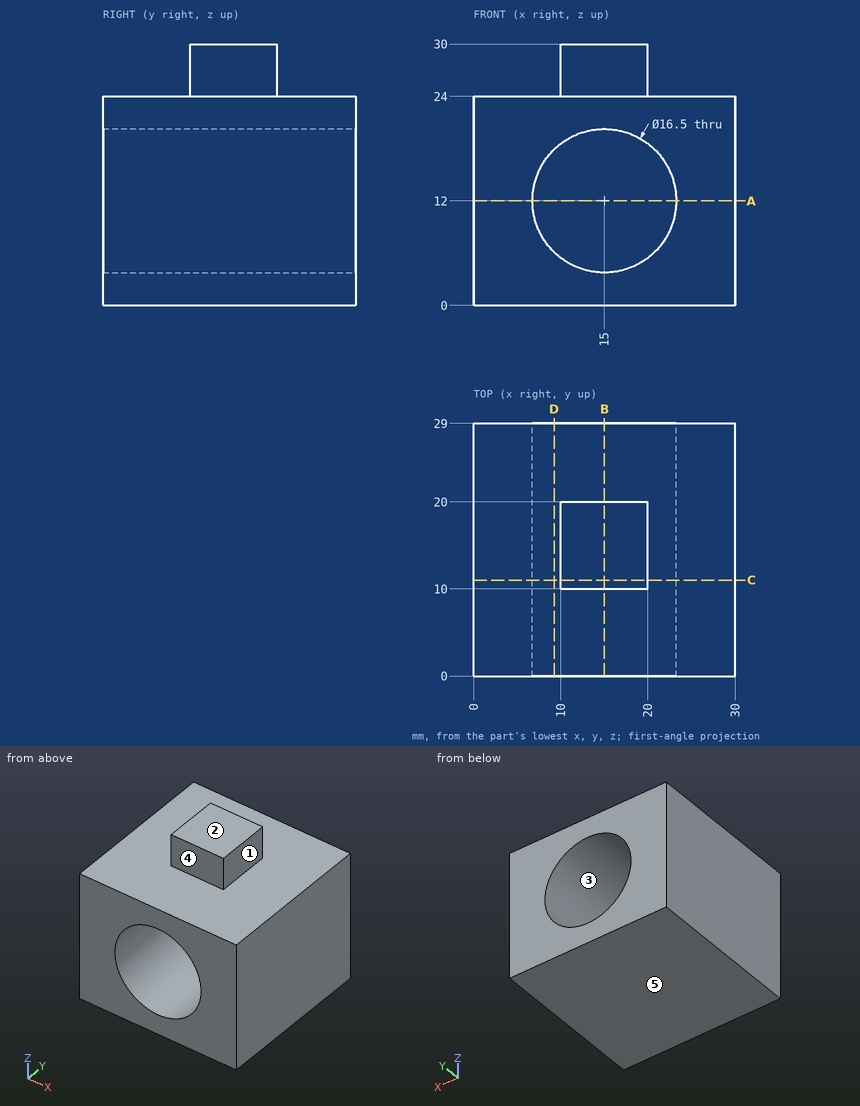
Geometry check sheet. Reference: drawing and pictorial views, mm from the part's lowest x, y, z. A direction names the side the tool comes from. Coordinates: 2 decimals unless noted, no trailing zeros. Loops run counter-clockwise (first coordinate to the right, second up) from the corner with the lowest first, then second, coordinate; pieces in that order, holes last. Notation, with made-up numbers: (0, 55.5) -> (53, 55.5) arc R30 cw to (53, 91.5) -> close; hole circle Ø1 at (12.5, 78). An arc over 180 degrees is marked (long way). Put each result on its own line as item: value.
1) Tool access check on the marked faces 1 and 2. Record the directions out of +Z, -Z, +X, -X, +Y, -Y that give a thin tool (end or side, any length) a straight path to the whole face; none if there is none.
Result set:
face 1: +Z, +X, +Y, -Y
face 2: +Z, +X, -X, +Y, -Y
2) Gauge pin test, flat ends, axial feed: pin 1 Ø1.8 at (y, z) = (17, 26) entering from -X; pin 2 Ø5 at (x, z) = (19.5, 14.5) entering from +Y; pin 3 Ø6.5 at (x, z) = (15.5, 27.5) entering from -Y; pin 4 Ø1.8 at (x, z) = (14, 27.5) entering from +Y. Record the tip position at first contact, or that the pin passes through.
Result set:
pin 1: stops at x = 10
pin 2: passes through
pin 3: stops at y = 10
pin 4: stops at y = 20
3) Thickness scan on line 1 (X direction, y = 23, z = 12); line 2 (X direction, y = 5.5, z = 18.75); line 3 (Z direction, x = 19.75, y = 27). Record the ranges inside material, lowest first.
Result set:
line 1: x = 0 to 6.75, 23.25 to 30
line 2: x = 0 to 10.26, 19.74 to 30
line 3: z = 0 to 5.25, 18.75 to 24
4) Cross-section at A-A on z = 12. Record the boundary of the cut face in (x, y), plus the area to 4 significant figures.
Result set:
outline: (0, 0) -> (6.75, 0) -> (6.75, 29) -> (0, 29) -> close; (23.25, 0) -> (30, 0) -> (30, 29) -> (23.25, 29) -> close
area: 391.5 mm^2
5) Cross-section at C-C on y = 11. Record the boundary of the cut face in (x, z).
Result set:
outline: (0, 0) -> (30, 0) -> (30, 24) -> (20, 24) -> (20, 30) -> (10, 30) -> (10, 24) -> (0, 24) -> close; hole circle Ø16.5 at (15, 12)
6) Release check for a two-part mould opening along Z. For the marked faces 3, 4 and 5 record: released by +Z, released by -Z, zero draft, split by the parting line, or undercut.
Result set:
face 3: undercut
face 4: zero draft
face 5: released by -Z
7) Cross-section at B-B on x = 15. Record the boundary of the cut face in (y, z), plus the area to 4 significant figures.
Result set:
outline: (0, 0) -> (29, 0) -> (29, 3.75) -> (0, 3.75) -> close; (0, 20.25) -> (29, 20.25) -> (29, 24) -> (20, 24) -> (20, 30) -> (10, 30) -> (10, 24) -> (0, 24) -> close
area: 277.5 mm^2
8) Cross-section at D-D on x = 9.25. Record the boundary of the cut face in (y, z), plus the area to 3 significant figures.
Result set:
outline: (0, 0) -> (29, 0) -> (29, 6.08) -> (0, 6.08) -> close; (0, 17.92) -> (29, 17.92) -> (29, 24) -> (0, 24) -> close
area: 353 mm^2
